from build123d import *

# Parameters (mm, degrees)
SKETCH2_R           = 50
SKETCH2_R_2         = 6
BOSS_EXTRUDE1_DEPTH = 40
CUT_EXTRUDE1_DEPTH  = 82.240384046
CIRPATTERN1_COUNT   = 6


with BuildPart() as part:
    # Sketch2 → Boss-Extrude1 (new body)
    with BuildSketch(Plane.XY):
        Circle(SKETCH2_R)
        Circle(SKETCH2_R_2, mode=Mode.SUBTRACT)
    extrude(amount=BOSS_EXTRUDE1_DEPTH)

    # Sketch1 → Cut-Extrude1 (cut, through all)
    with BuildSketch(Plane.XY.offset(40)):
        with BuildLine():
            Line((-5.543277195, -14.703899406), (-14.248413133, -35.719956649))
            ThreePointArc((-14.248413133, -35.719956649), (-14.036780749, -40.768068072), (-10.04438762, -43.864681434))
            ThreePointArc((-10.04438762, -43.864681434), (0, -45), (10.04438762, -43.864681434))
            ThreePointArc((10.04438762, -43.864681434), (14.036780749, -40.768068072), (14.248413133, -35.719956649))
            Line((14.248413133, -35.719956649), (5.543277195, -14.703899406))
            ThreePointArc((5.543277195, -14.703899406), (0, -11), (-5.543277195, -14.703899406))
        make_face()
    cut_extrude1 = extrude(amount=-CUT_EXTRUDE1_DEPTH, mode=Mode.SUBTRACT)

    # CirPattern1: Cut-Extrude1 ×6 about axis
    cirpattern1_axis = Axis((0, 0, 0), (0, 0, 1))
    for i in range(1, CIRPATTERN1_COUNT):
        add(cut_extrude1.rotate(cirpattern1_axis, i * 360 / CIRPATTERN1_COUNT), mode=Mode.SUBTRACT)

    # Sketch3 → Revolve1 (revolve)
    with BuildSketch(Plane(origin=(0, 0, 0), x_dir=(1, 0, 0), z_dir=(0, 1, 0))):
        with BuildLine():
            Line((50, 0), (50, -40))
            ThreePointArc((50, -40), (70, -20), (50, 0))
        make_face()
    revolve(axis=Axis((0, 0, 40), (0, 0, -1)))


solid = part.part
For this review, take the finished solid that the model builds, in its own axes (mm). Give positions to 0.01 mm unless a question says otherwise; leave off trailing zeros. Loops run counter-clockwise (first coordinate to the right, second up) from the corner with the lowest first, then second, coordinate; pieces in that order, holes last. Notation, with made-up numbers: (38.5, 85) -> (53.5, 85) arc R30 cw to (53.5, 114) -> close; hole circle Ø8 at (8.25, 8). An arc over 180 degrees is marked (long way). One line per question, with ' | ' between items.
1) We need section A-A (y = 0). Write out the cut boundary in (x, z), plus the area to 3 significant figures.
Resolved:
outline: (-50, 0) -> (-6, 0) -> (-6, 40) -> (-50, 40) arc R20 ccw to start; (6, 0) -> (50, 0) arc R20 ccw to (50, 40) -> (6, 40) -> close | area: 4,780 mm2
2) The part is to be moulded in two halves that separate along X. For faces 1 (the flat face through (10, 1, 40)), 2 (the cylindrical face through (-38.9, 22.62, 20.28)), say which applies: +X half, -X half, draft (parallel to the pull), parting line (faces both ways), or undercut.
Resolved:
face 1: draft | face 2: undercut
3) To check wall thickness, follow probe 1 along Y at (x, z) = (9.5, 19); probe 2 along Y at (x, z) = (-27.5, 35); probe 3 along Y at (x, z) = (12, 19). State the ranges of each line that lie inside material, in increasing order.
Resolved:
probe 1: y = -69.33 to -43.99, -24.26 to -11.45, -5.55 to 5.55, 11.45 to 24.26, 43.99 to 69.33 | probe 2: y = -56.94 to -32.45, -4.13 to 4.13, 32.45 to 56.94 | probe 3: y = -68.94 to -43.03, -30.29 to -14.81, -3.15 to 3.15, 14.81 to 30.29, 43.03 to 68.94
4) We need section C-C (y = -28.5). Give the number of separate pieces and of enclosed holes in the cut face, plus the area to 3 significant figures.
Resolved:
separate pieces: 4 | enclosed holes: 0 | area: 2,850 mm2
5) Insertion check: pin 1 Ø8 at (y, z) = (43.5, 29.5) entering from -X; pin 2 Ø2 at (x, y) = (19.5, -48.5) entering from -Z; pin 3 Ø2 at (x, y) = (-43.5, 46.5) entering from -Z. Each pin has a flat end and moves straight along its axis. Give the tip position at first contact, or say it passes through.
Resolved:
pin 1: stops at x = -55.64 | pin 2: stops at z = 0.04 | pin 3: stops at z = 4.53
6) We need section B-B (x = 0). Write out the cut boundary in (y, z), plus the area to 3 significant figures.
Resolved:
outline: (-50, 0) -> (-45, 0) -> (-45, 40) -> (-50, 40) arc R20 ccw to start; (-11, 0) -> (-6, 0) -> (-6, 40) -> (-11, 40) -> close; (6, 0) -> (11, 0) -> (11, 40) -> (6, 40) -> close; (45, 0) -> (50, 0) arc R20 ccw to (50, 40) -> (45, 40) -> close | area: 2,060 mm2
